Verification items for the finished model (mm, model axes). A direction names the side the tool comes from. Give positions to 0.01 mm unless a question says otherwise; leave off trailing zeros. Write each loop counter-clockwise with the first axis right and the second up, starting at its lowest first coordinate (ties: lowest second). Pieces come first, ordered by that corner, then holes. Notation, with made-up numbers: (-27.5, 86) -> (-4.5, 86) arc R13 cw to (-4.5, 94) -> close; hole circle Ø11 at (-19.5, 60). An arc over 180 degrees is marked (long way). Answer as CSV lines item,"result".
```python
from build123d import *

# Parameters (mm, degrees)
SKETCH1_W           = 115
SKETCH1_H           = 140
BOSS_EXTRUDE1_DEPTH = 2.4
CUT_EXTRUDE1_DEPTH  = 3.4
FILLET1_R           = 10
SKETCH3_W           = 2.4
SKETCH3_H           = 140
BOSS_EXTRUDE2_DEPTH = 25
FILLET2_R           = 10
SKETCH4_R           = 2.75
CUT_EXTRUDE2_DEPTH  = 116
SKETCH5_R           = 14.26
SKETCH5_R_2         = 2.75
CUT_EXTRUDE3_DEPTH  = 3.4
SKETCH6_R           = 3.375
CUT_EXTRUDE4_DEPTH  = 116


with BuildPart() as part:
    # Sketch1 → Boss-Extrude1 (new body)
    with BuildSketch(Plane(origin=(0, 0, 0), x_dir=(0, 0, -1), z_dir=(1, 0, 0))):
        with Locations((57.5, -70)):
            Rectangle(SKETCH1_W, SKETCH1_H)
    extrude(amount=BOSS_EXTRUDE1_DEPTH)

    # Sketch2 → Cut-Extrude1 (cut, through all)
    with BuildSketch(Plane(origin=(2.4, 0, 0), x_dir=(0, 0, -1), z_dir=(1, 0, 0))):
        Polygon((87, 0), (115, -30), (142.616199658, -32.505405645), (142.616199658, 14.875556406), align=None)
        Polygon((115, -110), (87, -140), (87, -152.661109726), (136.310004643, -152.661109726), align=None)
    extrude(amount=-CUT_EXTRUDE1_DEPTH, mode=Mode.SUBTRACT)

    # Fillet1
    fillet1_edges = [part.edges().sort_by_distance(p)[0] for p in [
        (1.2, 0, -87),
        (1.2, -30, -115),
        (1.2, -110, -115),
        (1.2, -140, -87),
    ]]
    fillet(fillet1_edges, radius=FILLET1_R)

    # Sketch3 → Boss-Extrude2 (add)
    with BuildSketch(Plane(origin=(2.4, 0, 0), x_dir=(0, 0, -1), z_dir=(1, 0, 0))):
        with Locations((1.2, -70)):
            Rectangle(SKETCH3_W, SKETCH3_H)
    extrude(amount=BOSS_EXTRUDE2_DEPTH)

    # Fillet2
    fillet2_edges = [part.edges().sort_by_distance(p)[0] for p in [
        (27.4, -140, -1.2),
        (27.4, 0, -1.2),
    ]]
    fillet(fillet2_edges, radius=FILLET2_R)

    # Sketch4 → Cut-Extrude2 (cut, through all)
    with BuildSketch(Plane.XY):
        with Locations((11.974983581, -70)):
            Circle(SKETCH4_R)
        with Locations((11.974983581, -25)):
            Circle(SKETCH4_R)
        with Locations((11.974983581, -115)):
            Circle(SKETCH4_R)
    extrude(amount=-CUT_EXTRUDE2_DEPTH, mode=Mode.SUBTRACT)

    # Sketch5 → Cut-Extrude3 (cut, through all)
    with BuildSketch(Plane(origin=(2.4, 0, 0), x_dir=(0, 0, -1), z_dir=(1, 0, 0))):
        with Locations((89.027947804, -96.494029199)):
            Circle(SKETCH5_R)
        with Locations((77.277947804, -76.14243221)):
            Circle(SKETCH5_R_2)
        with Locations((100.777947804, -76.14243221)):
            Circle(SKETCH5_R_2)
        with Locations((100.777947804, -116.845626188)):
            Circle(SKETCH5_R_2)
        with Locations((77.277947804, -116.845626188)):
            Circle(SKETCH5_R_2)
        with Locations((65.527947804, -96.494029199)):
            Circle(SKETCH5_R_2)
    extrude(amount=-CUT_EXTRUDE3_DEPTH, mode=Mode.SUBTRACT)

    # Sketch6 → Cut-Extrude4 (cut, through all)
    with BuildSketch(Plane.XY):
        with Locations((12.4, -105)):
            Circle(SKETCH6_R)
    extrude(amount=-CUT_EXTRUDE4_DEPTH, mode=Mode.SUBTRACT)


solid = part.part
```
1) Depth check by flat-ended pin: pin 1 (12 mm diameter, centred on x = 3, z = -98.5, fed in from +Y); pin 2 (12 mm diameter, centred on y = -19, z = -34.5, fed in from +X). Enter the tip coordinate at first touch or a pass-through.
Reported:
pin 1,"y = -5.93"
pin 2,"x = 2.4"
2) Scan lines: line 1 along Z through (x, y) = (15.5, -69.5); line 2 along X through (y, z) = (-113, -25). Record each from-to range of solid material in increasing order.
Reported:
line 1,"-2.4 to 0"
line 2,"0 to 2.4"
3) Tool access check on faces 5 (the flat face through (15, -71, -2.4)), 6 (the flat face through (2, 0, -35)). Record the directions out of +Z, -Z, +X, -X, +Y, -Y that give a thin tool (end or side, any length) a straight path to the whole face; none if there is none.
Reported:
face 5,"-Z, +X, +Y, -Y"
face 6,"+Z, -Z, +X, -X, +Y"
4) Section check C-C (x = 12.4). Record the boundary of the cut face in (y, z) (3 decimals), and give its area (3 significant figures).
Reported:
outline,"(-140, -2.4) -> (-117.717, -2.4) -> (-117.717, 0) -> (-140, 0) -> close; (-112.283, -2.4) -> (-108.375, -2.4) -> (-108.375, 0) -> (-112.283, 0) -> close; (-101.625, -2.4) -> (-72.717, -2.4) -> (-72.717, 0) -> (-101.625, 0) -> close; (-67.283, -2.4) -> (-27.717, -2.4) -> (-27.717, 0) -> (-67.283, 0) -> close; (-22.283, -2.4) -> (0, -2.4) -> (0, 0) -> (-22.283, 0) -> close"
area,"281 mm²"
5) Draft check along Y on faces 1 (the cylindrical face through (9.95, -23.14, -1.18)), 2 (the cylindrical face through (1.22, -75.32, -103.4)), 3 (the cylindrical face through (1.183, -139.194, -86.587)), 4 (the flat face through (0, -69, -57)). Enter one of: +Y half, -Y half, draft (parallel to the pull), parting line (faces both ways), or undercut.
Reported:
face 1,"undercut"
face 2,"undercut"
face 3,"-Y half"
face 4,"draft"
6) Section check B-B (y = -25). Record the boundary of the cut face in (x, z), and give its area (3 significant figures).
Reported:
outline,"(0, -110.33) -> (2.4, -110.33) -> (2.4, -2.4) -> (9.22, -2.4) -> (9.22, 0) -> (0, 0) -> close; (14.72, -2.4) -> (27.4, -2.4) -> (27.4, 0) -> (14.72, 0) -> close"
area,"312 mm²"
7) Section check D-D (y = -122). Record the boundary of the cut face in (x, z), and give its area (3 significant figures).
Reported:
outline,"(0, -103.8) -> (2.4, -103.8) -> (2.4, -2.4) -> (27.4, -2.4) -> (27.4, 0) -> (0, 0) -> close"
area,"309 mm²"
8) Section check A-A (z = -96). Record the boundary of the cut face in (x, y), and give its area (3 significant figures).
Reported:
outline,"(0, -130.36) -> (2.4, -130.36) -> (2.4, -108.93) -> (0, -108.93) -> close; (0, -84.05) -> (2.4, -84.05) -> (2.4, -9.64) -> (0, -9.64) -> close"
area,"230 mm²"
